```python
from build123d import *

# Parameters (mm, degrees)
SKETCH2_W           = 5.99
SKETCH2_H           = 5.99
BOSS_EXTRUDE1_DEPTH = 3.6
SKETCH3_R           = 1.75
BOSS_EXTRUDE2_DEPTH = 1.4
FILLET1_R           = 0.15
SKETCH5_R           = 0.6
BOSS_EXTRUDE3_DEPTH = 0.4


with BuildPart() as part:
    # Sketch2 → Boss-Extrude1 (new body)
    with BuildSketch(Plane.XY):
        with Locations((2.995, 2.995)):
            Rectangle(SKETCH2_W, SKETCH2_H)
    extrude(amount=BOSS_EXTRUDE1_DEPTH)

    # Sketch3 → Boss-Extrude2 (add)
    with BuildSketch(Plane.XY.offset(3.6)):
        with Locations(Location((2.995, 2.995, 0), (0, 0, 180))):
            Circle(SKETCH3_R)
    extrude(amount=BOSS_EXTRUDE2_DEPTH)

    # Fillet1
    fillet1_edges = [part.edges().sort_by_distance(p)[0] for p in [
        (4.745, 2.995, 5),
        (0, 5.99, 1.8),
        (5.99, 5.99, 1.8),
        (5.99, 0, 1.8),
        (0, 0, 1.8),
    ]]
    fillet(fillet1_edges, radius=FILLET1_R)

    # Sketch5 → Boss-Extrude3 (add)
    with BuildSketch(Plane.XY.offset(3.6)):
        with Locations(Location((1.105, 4.88, 0), (0, 0, 180))):
            Circle(SKETCH5_R)
        with Locations(Location((4.885, 4.88, 0), (0, 0, 180))):
            Circle(SKETCH5_R)
        with Locations(Location((4.885, 1.11, 0), (0, 0, 180))):
            Circle(SKETCH5_R)
        with Locations(Location((1.105, 1.11, 0), (0, 0, 180))):
            Circle(SKETCH5_R)
    extrude(amount=BOSS_EXTRUDE3_DEPTH)


solid = part.part
```
Geometry check sheet. Reference: the model listing, model coordinates, mm. A direction names the side the tool comes from. Round coordinates to 2 decimals unless told otherwise and drop trailing zeros. Order: outer loops, then holes, each group sorted by start corner. A loop starts at its lowest first (then second) coordinate and runs counter-clockwise, first axis right, second up. Notation, with made-up numbers: M 16,27 L 47,27 A24 ccw 47,55 Z; hole C -36.5,60 d6. An arc over 180 degrees is marked long. Write item = value, one per line.
Q1. Set-up check for faces 4 (the flat face through (1.6, 1.7, 3.6)), 5 (the flat face through (5, 5, 4)), 6 (the flat face through (5, 1, 4)): record each of +Z, -Z, +X, -X, +Y, -Y from which the full face is reachable in a straight line by a thin tool's end or side.
Answer block:
face_4 = +Z
face_5 = +Z, +X, +Y
face_6 = +Z, +X, -Y
Q2. Scan lines: line 1 (Z direction, x = 3.85, y = 1.05); line 2 (X direction, y = 4.8, z = 3.85); line 3 (Z direction, x = 1.25, y = 0.95). Record each from-to range of solid material in increasing order.
Answer block:
line_1 = 0 to 3.6
line_2 = 0.51 to 1.7, 4.29 to 5.48
line_3 = 0 to 4
Q3. Section check D-D (z = 4.7). Enter the section's corners in (x, y) (3 decimals).
Answer block:
outline = C 2.995,2.995 d3.5
Q4. Release check for a two-part mould opening along X. For faces 1 (the cylindrical face through (1.547, 4.474, 3.797)), 2 (the flat face through (1, 1, 4)), 3 (the flat face through (0, 3, 2)) record: released by +X, released by -X, zero draft, split by the parting line, or undercut.
Answer block:
face_1 = undercut
face_2 = zero draft
face_3 = released by -X
Q5. Section check B-B (x = 5.05). Enter the section's corners in (y, z), plus the area to 3 significant figures.
Answer block:
outline = M 0,0 L 5.99,0 L 5.99,3.6 L 5.46,3.6 L 5.46,4 L 4.3,4 L 4.3,3.6 L 1.69,3.6 L 1.69,4 L 0.53,4 L 0.53,3.6 L 0,3.6 Z
area = 22.5 mm^2
Q6. Section check C-C (x = 5.65). Enter the section's corners in (y, z).
Answer block:
outline = M 0,0 L 5.99,0 L 5.99,3.6 L 0,3.6 Z
Q7. Depth check by flat-ended pin: pin 1 Ø1.5 at (x, y) = (3, 4.5) entering from -Z; pin 2 Ø1 at (x, y) = (5, 1) entering from +Z. Enter the tip coordinate at first touch or a pass-through.
Answer block:
pin_1 = 0
pin_2 = 4
Q8. Section check A-A (y = 4.88). Enter the section's corners in (x, z) (3 decimals).
Answer block:
outline = M 0,0 L 5.99,0 L 5.99,3.6 L 5.485,3.6 L 5.485,4 L 4.285,4 L 4.285,3.6 L 1.705,3.6 L 1.705,4 L 0.505,4 L 0.505,3.6 L 0,3.6 Z
